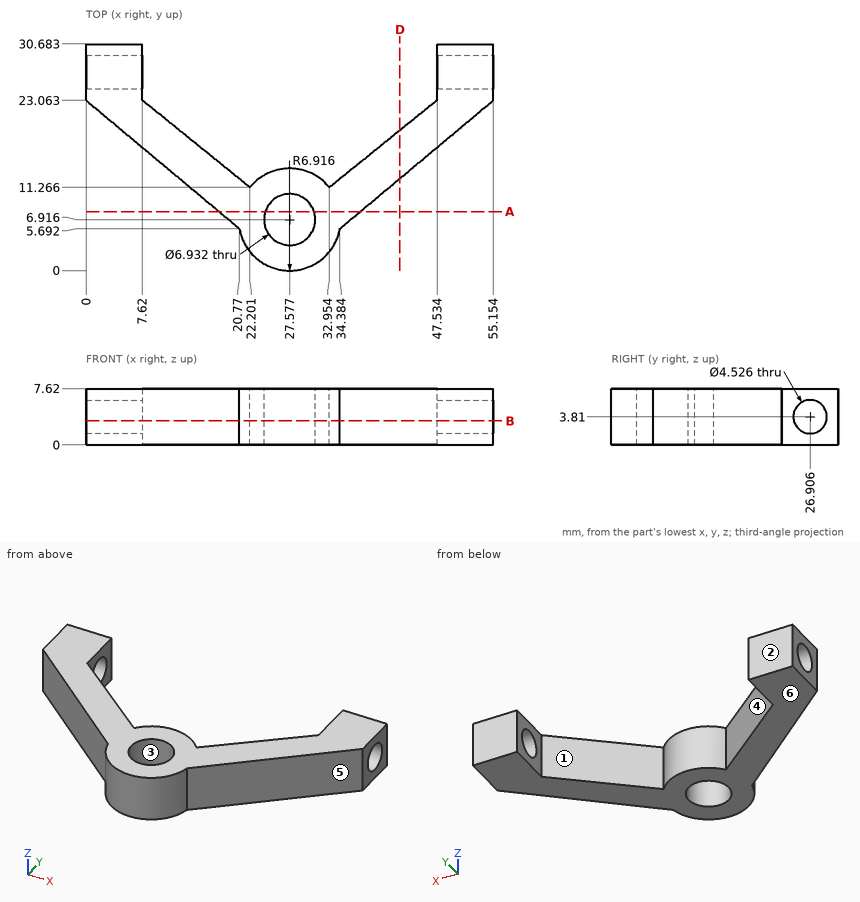
Answer from the drawing. Dimensions are ordinates in mm from the lowest x, y and z of the part. A direction names the side the tool comes from. Give positions to 0.01 mm unless a question says otherwise; leave off trailing zeros. Write each loop counter-clockwise with the first axis right and the second up, starting at its lowest first coordinate (ties: lowest second). Pieces come first, ordered by that corner, then holes. Notation, with made-up numbers: (83.25, -33) -> (130.25, -33) arc R14 ccw to (130.25, -28) -> close; hole circle Ø2 at (31, 63.5). An arc over 180 degrees is marked (long way). Use a Markdown table: item, result.
(1) Determine the mould class of the marked faces 3, 4, 5 and 6 for opening direction X: released by +X, released by -X, zero draft, split by the parting line, or undercut.
Return value:
| item | result |
|---|---|
| face 3 | undercut |
| face 4 | undercut |
| face 5 | released by +X |
| face 6 | zero draft |
(2) Flat-ended cylindrical pins translate along their axes: P1, Ø2.5, axis at y = 26.5, z = 3, coming from the +X side; P2, Ø1, axis at y = 22.5, z = 4, coming from the +X side; P3, Ø3, axis at x = 18.5, z = 3, coming from the +Y side (1 decimal). Find the tip coordinate at first contact, or state that the pin passes through.
Return value:
| item | result |
|---|---|
| P1 | through |
| P2 | x = 55.08 |
| P3 | y = 15.5 |
(3) Section A-A, the plane y = 8 is taken. Determine the outline of the cut face in (x, z) (1 decimal).
Return value:
| item | result |
|---|---|
| outline | (18, 0) -> (24.3, 0) -> (24.3, 7.6) -> (18, 7.6) -> close; (30.9, 0) -> (37.1, 0) -> (37.1, 7.6) -> (30.9, 7.6) -> close |
(4) Section B-B, the plane z = 3.25 is taken. Determine the outline of the cut face in (x, y) (1 decimal).
Return value:
| item | result |
|---|---|
| outline | (0, 23.1) -> (20.8, 5.7) arc R6.9 ccw to (34.4, 5.7) -> (55.2, 23.1) -> (55.2, 24.7) -> (47.5, 24.7) -> (47.5, 23.1) -> (33, 11.3) arc R6.9 ccw to (22.2, 11.3) -> (7.6, 23.1) -> (7.6, 24.7) -> (0, 24.7) -> close; (0, 29.1) -> (7.6, 29.1) -> (7.6, 30.7) -> (0, 30.7) -> close; (47.5, 29.1) -> (55.2, 29.1) -> (55.2, 30.7) -> (47.5, 30.7) -> close; hole circle Ø6.9 at (27.6, 6.9) |
(5) For the marked faces 1 and 2, determine the directions among +Z, -Z, +X, -X, +Y, -Y from which every point of the face is accessible in a straight line to the end or side of a thin tool.
Return value:
| item | result |
|---|---|
| face 1 | +Z, -Z, +Y |
| face 2 | +Z, -Z, +X, -X, +Y |
(6) Section D-D, the plane x = 42.5 is taken. Determine the outline of the cut face in (y, z), then the cut area to 3 significant figures.
Return value:
| item | result |
|---|---|
| outline | (12.48, 0) -> (18.99, 0) -> (18.99, 7.62) -> (12.48, 7.62) -> close |
| area | 49.6 mm2 |
(7) Find the intervals of material crossed by probe 1 along X at (y, z) = (24.5, 1.75) (1 decimal); probe 2 along Z at (x, y) = (4, 27); probe 3 along X at (y, z) = (21, 4.5) (1 decimal), in increasing order. Write a range as from..to.
Return value:
| item | result |
|---|---|
| probe 1 | 0..7.6, 47.5..55.2 |
| probe 2 | 0..1.55, 6.07..7.62 |
| probe 3 | 2.5..10.2, 45..52.7 |
